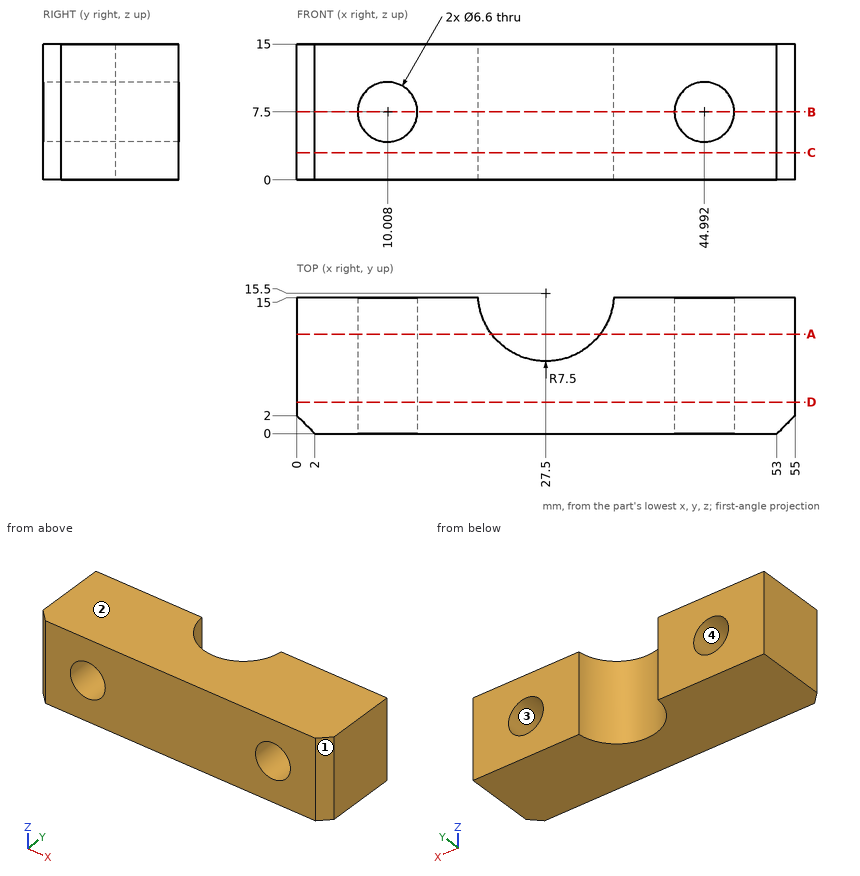
Input: dimensioned drawing with shaded views. Units: mm. Origin: part minimum x, y, z. Coordinates: 2 decimals unless noted, no trailing zeros. Order: outer loops, then holes, each group sorted by start corner. A loop starts at its lowest first (then second) coordinate and runs counter-clockwise, first axis right, second up.
(1) Section query C-C (z = 3). Return the cut outline in (x, y).
(2) Section query A-A (y = 11). Return the cut outline in (x, z).
(3) Section query B-B (z = 7.5). Return the cut outline in (x, y), plus the area to 3 significant figures.
(4) First-contact query: pin 1 (5.5 mm diameter, centred on x = 10.01, z = 7.5, fed in from -Y). Flat tip, straight axial feed; report the tip coordinate or a pass-through.
(5) Draft query along Z for the marked faces 1, 2, 3 and 4. Return one class per face: pulls with the +Z half, pulls with the -Z half, needs draft (parallel to the pull), parting line crosses it, or undercut.
(6) Material intervals for probe 1 along X at (y, z) = (11, 5) (1 decimal); probe 2 along X at (y, z) = (10.25, 7) (1 decimal); probe 3 along X at (y, z) = (2.5, 9.5) (1 decimal), sorted ascending.
(7) Section query D-D (y = 3.5). Return the cut outline in (x, z).
Solution:
1. outline: (0, 2) - (2, 0) - (53, 0) - (55, 2) - (55, 15) - (34.98, 15) arc R7.5 cw to (20.02, 15) - (0, 15) - close
2. outline: (0, 0) - (21.5, 0) - (21.5, 15) - (0, 15) - close; (33.5, 0) - (55, 0) - (55, 15) - (33.5, 15) - close; hole circle Ø6.6 at (10.01, 7.5); hole circle Ø6.6 at (44.99, 7.5)
3. outline: (0, 2) - (2, 0) - (6.71, 0) - (6.71, 15) - (0, 15) - close; (13.31, 0) - (41.69, 0) - (41.69, 15) - (34.98, 15) arc R7.5 cw to (20.02, 15) - (13.31, 15) - close; (48.29, 0) - (53, 0) - (55, 2) - (55, 15) - (48.29, 15) - close
3. area: 542 mm2
4. pin 1: passes through
5. face 1: needs draft
5. face 2: pulls with the +Z half
5. face 3: undercut
5. face 4: undercut
6. probe 1: x = 0 to 7.9, 12.2 to 21.5, 33.5 to 42.8, 47.1 to 55
6. probe 2: x = 0 to 6.7, 13.3 to 22.1, 32.9 to 41.7, 48.3 to 55
6. probe 3: x = 0 to 7.4, 12.6 to 42.4, 47.6 to 55
7. outline: (0, 0) - (55, 0) - (55, 15) - (0, 15) - close; hole circle Ø6.6 at (10.01, 7.5); hole circle Ø6.6 at (44.99, 7.5)
